from build123d import *

# Parameters (mm, degrees)
SKETCH003_R        = 4.5
PAD001_DEPTH       = 14
POLARPATTERN_COUNT = 4
SKETCH004_R        = 3.5
PAD002_DEPTH       = 1.5
SKETCH005_R        = 3.5
PAD003_DEPTH       = 23
SKETCH011_R        = 7.5
PAD007_DEPTH       = 8
POCKET004_DEPTH    = 3.5


with BuildPart() as part:
    # Sketch003 → Pad001 (new body)
    with BuildSketch(Plane.XY):
        Circle(SKETCH003_R)
        with BuildLine():
            Line((-1.5, 17.5), (-1.5, -17.5))
            ThreePointArc((-1.5, -17.5), (0, -19), (1.5, -17.5))
            Line((1.5, -17.5), (1.5, 17.5))
            ThreePointArc((1.5, 17.5), (0, 19), (-1.5, 17.5))
        make_face()
    pad001 = extrude(amount=PAD001_DEPTH)

    # PolarPattern: Pad001 ×4 about axis
    polarpattern_axis = Axis((0, 0, 0), (0, 0, 1))
    for i in range(1, POLARPATTERN_COUNT):
        add(pad001.rotate(polarpattern_axis, i * 360 / POLARPATTERN_COUNT))

    # Sketch004 (on Face17 of MultiTransform) → Pad002 (join)
    with BuildSketch(Plane(origin=(0, 0, 0), x_dir=(1, 0, 0), z_dir=(0, 0, -1))):
        Circle(SKETCH004_R)
    extrude(amount=PAD002_DEPTH)

    # Sketch005 (on Face4 of Pad002) → Pad003 (join)
    with BuildSketch(Plane.XY.offset(14)):
        Circle(SKETCH005_R)
    extrude(amount=PAD003_DEPTH)

    # Sketch011 (on Face22 of Pad003) → Pad007 (join)
    with BuildSketch(Plane.XY.offset(37)):
        Circle(SKETCH011_R)
    extrude(amount=PAD007_DEPTH)

    # Sketch012 (on Face24 of Pad007) → Pocket004 (cut)
    with BuildSketch(Plane.XY.offset(45)):
        with BuildLine():
            ThreePointArc((2.645751, 3), (-4, 0), (2.645751, -3))
            Line((2.645751, -3), (10.145751, -3))
            Line((10.145751, -3), (10.145751, 3))
            Line((10.145751, 3), (2.645751, 3))
        make_face()
    extrude(amount=-POCKET004_DEPTH, mode=Mode.SUBTRACT)


solid = part.part
Read the model definition and answer for the solid it produces. Units are mm, in the model's axes. A direction names the side the tool comes from. Round coordinates to 2 decimals unless told otherwise and drop trailing zeros. Write each loop counter-clockwise with the first axis right and the second up, starting at its lowest first coordinate (ties: lowest second). Pieces come first, ordered by that corner, then holes. Notation, with made-up numbers: M 33.5,59.25 L 57.5,59.25 A12 ccw 57.5,63.25 Z; hole C 48.5,-3.75 d11. An arc over 180 degrees is marked long. Use a Markdown table: item, result.
1) The part is cut by section D-D (z = 32). Write down the section's boundary in (x, y).
Answers follow:
| item | result |
|---|---|
| outline | C 0,0 d7 |
2) A tool of negligible diameter and unlimited length cuts with its end or side. For faces 1 (the flat face through (-11, 1.5, 7)), 2 (the flat face through (1.5, -11, 7)), 3 (the cylindrical face through (3.233, -1.341, 25.339)), 4 (the flat face through (5, 3, 43)), 5 (the flat face through (-3, -3, 0)), from which of +Z, -Z, +X, -X, +Y, -Y can it reach the whole face along a straight path? Write none if from no direction.
Answers follow:
| item | result |
|---|---|
| face 1 | -Z, -X, +Y |
| face 2 | -Z, +X, -Y |
| face 3 | none |
| face 4 | +Z, +X |
| face 5 | -Z |
3) For a pull along Y with two mould halves and no side action, classify faces 6 (the cylindrical face through (3.233, 1.341, -0.74)), 7 (the flat face through (5, -3, 43)), 8 (the flat face through (-3, -3, 14)) as pulls with the +Y half, pulls with the -Y half, needs draft (parallel to the pull), parting line crosses it, or undercut.
Answers follow:
| item | result |
|---|---|
| face 6 | parting line crosses it |
| face 7 | undercut |
| face 8 | needs draft |
4) The part is cut by section B-B (x = 0). Write down the section's boundary in (y, z).
Answers follow:
| item | result |
|---|---|
| outline | M -19,0 L -3.5,0 L -3.5,-1.5 L 3.5,-1.5 L 3.5,0 L 19,0 L 19,14 L 3.5,14 L 3.5,37 L 7.5,37 L 7.5,45 L 4,45 L 4,41.5 L -4,41.5 L -4,45 L -7.5,45 L -7.5,37 L -3.5,37 L -3.5,14 L -19,14 Z |
5) The part is cut by section C-C (y = 9.5). Write down the section's boundary in (x, z), plus the area to 3 significant figures.
Answers follow:
| item | result |
|---|---|
| outline | M -1.5,0 L 1.5,0 L 1.5,14 L -1.5,14 Z |
| area | 42.0 mm2 |
6) Flat-ended cylindrical pins translate along their axes: pin 1 (3 mm diameter, centred on x = 7, y = -1, fed in from +Z); pin 2 (2 mm diameter, centred on x = 11, z = 8, fed in from +Y); pin 3 (5 mm diameter, centred on x = -10, y = -3.5, fed in from +Z); pin 4 (12 mm diameter, centred on x = 9.5, y = 11.5, fed in from -Z). Find the tip coordinate at first contact, or state that the pin passes through.
Answers follow:
| item | result |
|---|---|
| pin 1 | stops at z = 41.5 |
| pin 2 | stops at y = 1.5 |
| pin 3 | stops at z = 14 |
| pin 4 | passes through |
7) Straight lines are drawn through the part: line 1 along Y through (x, z) = (0, 43.25); line 2 along Z through (x, y) = (-3, -2.5); line 3 along X through (y, z) = (0, 42.3). For each, find the intervals that lie inside material, in ascending order. Write a range as [from, to].
Answers follow:
| item | result |
|---|---|
| line 1 | y = [-7.5, -4], [4, 7.5] |
| line 2 | z = [0, 14], [37, 41.5] |
| line 3 | x = [-7.5, -4] |
8) The part is cut by section A-A (z = 5.5). Write down the section's boundary in (x, y).
Answers follow:
| item | result |
|---|---|
| outline | M -17.5,-1.5 L -4.24,-1.5 A4.5 ccw -1.5,-4.24 L -1.5,-17.5 A1.5 ccw 1.5,-17.5 L 1.5,-4.24 A4.5 ccw 4.24,-1.5 L 17.5,-1.5 A1.5 ccw 17.5,1.5 L 4.24,1.5 A4.5 ccw 1.5,4.24 L 1.5,17.5 A1.5 ccw -1.5,17.5 L -1.5,4.24 A4.5 ccw -4.24,1.5 L -17.5,1.5 A1.5 ccw Z |
